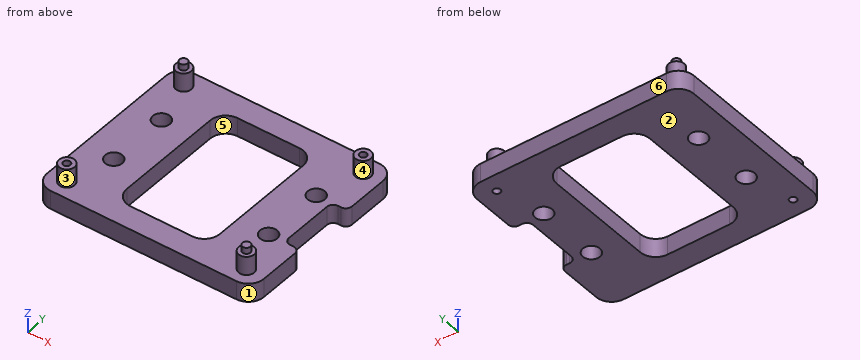
```python
from build123d import *

# Parameters (mm, degrees)
F0_R     = 1.15
F0_R_2   = 2.75
F0_W     = 30
F0_H     = 45
F1_DEPTH = 6
F2_R     = 5
F4_R     = 2.5
F5_DEPTH = 6
F3_R     = 1.3
F6_DEPTH = 8
F7_R     = 1.15
F8_DEPTH = 25
F9_R     = 2


# Not quite as in the source:
# - a feature names something its author has since deleted; it is built from what else it names


with BuildPart() as f1:
    # F0 (on Top) → F1 (new body)
    with BuildSketch(Plane.XY):
        Polygon((35, 30), (-35, 30), (-35, -30), (35, -30), (35, -10), (30, -10), (30, 10), (35, 10), align=None)
        with Locations((-29, -24.5)):
            Circle(F0_R, mode=Mode.SUBTRACT)
        with Locations((-25, -10)):
            Circle(F0_R_2, mode=Mode.SUBTRACT)
        with Locations((25, -10)):
            Circle(F0_R_2, mode=Mode.SUBTRACT)
        with Locations((-25, 10)):
            Circle(F0_R_2, mode=Mode.SUBTRACT)
        Rectangle(F0_W, F0_H, mode=Mode.SUBTRACT)
        with Locations((25, 10)):
            Circle(F0_R_2, mode=Mode.SUBTRACT)
        with Locations((29, 24.5)):
            Circle(F0_R, mode=Mode.SUBTRACT)
    extrude(amount=F1_DEPTH)

    # F2
    f2_edges = [f1.edges().sort_by_distance(p)[0] for p in [
        (-35, -30, 3),
        (-35, 30, 3),
        (-15, 22.5, 3),
        (15, 22.5, 3),
        (15, -22.5, 3),
        (-15, -22.5, 3),
        (35, 30, 3),
        (35, -30, 3),
    ]]
    fillet(f2_edges, radius=F2_R)

    # F4 (on face) → F5 (join)
    with BuildSketch(Plane.XY.offset(6)):
        with Locations((-29, 24.5)):
            Circle(F4_R)
        with Locations((29, 24.5)):
            Circle(F4_R)
        with Locations((29, -24.5)):
            Circle(F4_R)
        with Locations((-29, -24.5)):
            Circle(F4_R)
    extrude(amount=F5_DEPTH)

    # F3 (on face) → F6 (join)
    with BuildSketch(Plane.XY.offset(6)):
        with Locations((-29, 24.5)):
            Circle(F3_R)
        with Locations((29, -24.5)):
            Circle(F3_R)
    extrude(amount=F6_DEPTH)

    # F7 (on face) → F8 (cut)
    with BuildSketch(Plane.XY.offset(12)):
        with Locations((-29, -24.5)):
            Circle(F7_R)
        with Locations((29, 24.5)):
            Circle(F7_R)
    extrude(amount=-F8_DEPTH, mode=Mode.SUBTRACT)

    # F9
    f9_edges = [f1.edges().sort_by_distance(p)[0] for p in [
        (35, 10, 3),
        (30, 10, 3),
        (30, -10, 3),
        (35, -10, 3),
    ]]
    fillet(f9_edges, radius=F9_R)


solid = f1.part
```
Work out the finished part from the listing and answer in its coordinate system (mm). Face numbers are marked on the shaded views. A direction names the side the tool comes from. Coordinates: 2 decimals unless noted, no trailing zeros. Loops run counter-clockwise (first coordinate to the right, second up) from the corner with the lowest first, then second, coordinate; pieces in that order, holes last.
1) Section A-A (y = -4.5) is taken. Give the vertices of the cut face in (x, z).
Results:
outline: (-35, 0) - (-15, 0) - (-15, 6) - (-35, 6) - close; (15, 0) - (30, 0) - (30, 6) - (15, 6) - close
2) Section B-B (x = -29) is taken. Give the vertices of the cut face in (y, z), plus the area to 3 significant figures.
Results:
outline: (-30, 0) - (-25.65, 0) - (-25.65, 12) - (-27, 12) - (-27, 6) - (-30, 6) - close; (-23.35, 0) - (30, 0) - (30, 6) - (27, 6) - (27, 12) - (25.8, 12) - (25.8, 14) - (23.2, 14) - (23.2, 12) - (22, 12) - (22, 6) - (-22, 6) - (-22, 12) - (-23.35, 12) - close
area: 398 mm2
3) Section D-D (x = 13) is taken. Give the vertices of the cut face in (y, z), plus the area to 3 significant figures.
Results:
outline: (-30, 0) - (-21.5, 0) - (-21.5, 6) - (-30, 6) - close; (21.5, 0) - (30, 0) - (30, 6) - (21.5, 6) - close
area: 102 mm2
4) For a pull along X with two mould halves and no side action, classify the marked faces 1, 2 and 3 as +X half, -X half, draft (parallel to the pull), parting line (faces both ways), or undercut.
Results:
face 1: +X half
face 2: draft
face 3: undercut
5) Consider probe 1 along Y at (x, z) = (-25, 4.6); probe 2 along X at (y, z) = (14, 5); probe 3 along Y at (x, z) = (2, 3.25). Determine where each line is inside the solid, lowest interval first.
Results:
probe 1: y = -30 to -12.75, -7.25 to 7.25, 12.75 to 30
probe 2: x = -35 to -15, 15 to 35
probe 3: y = -30 to -22.5, 22.5 to 30
6) Flat-ended cylindrical pins translate along their axes: pin 1 (5 mm diameter, centred on y = -1.5, z = 3.5, fed in from +X); pin 2 (7 mm diameter, centred on x = -25, y = -10, fed in from +Z); pin 3 (5.5 mm diameter, centred on x = -30, y = -24.5, fed in from +Z). Find the tip coordinate at first contact, or state that the pin passes through.
Results:
pin 1: stops at x = 30
pin 2: stops at z = 6
pin 3: stops at z = 12
7) Section C-C (z = 4) is taken. Give the number of separate pieces and of enclosed holes in the cut face, plus the area to 3 significant figures.
Results:
separate pieces: 1
enclosed holes: 7
area: 2,650 mm2
8) For the marked faces 4, 5 and 6, determine the directions among +Z, -Z, +X, -X, +Y, -Y from which every point of the face is accessible in a straight line to the end or side of a thin tool.
Results:
face 4: +Z
face 5: +Z, -Z
face 6: +Z, -Z, +X, -X, +Y
